For this review, take the finished solid that the model builds, in its own axes (mm). Face numbers are marked on the shaded views. A direction names the side the tool comes from. Give positions to 0.01 mm unless a question says otherwise; leave off trailing zeros. Write each loop counter-clockwise with the first axis right and the second up, starting at its lowest first coordinate (ties: lowest second). Pieces come first, ordered by that corner, then holes. Notation, with made-up numbers: (-37.5, 3) -> (17.5, 3) arc R26 ccw to (17.5, 41) -> close; hole circle Ø6 at (43, 84). An arc over 180 degrees is marked (long way). Return JSON: item names as keys, results as strings.
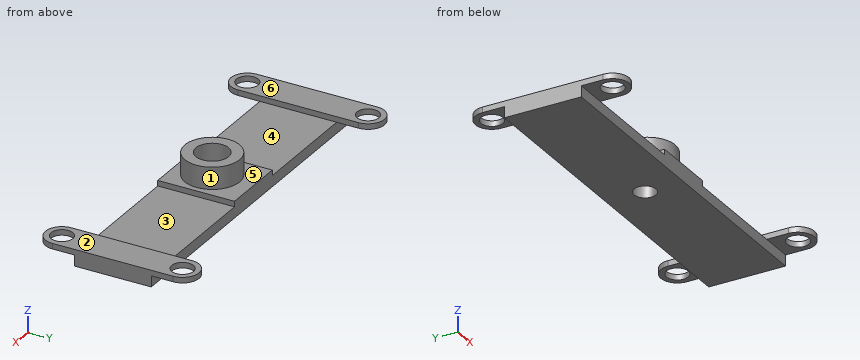
from build123d import *

# Parameters (mm, degrees)
ESBO_O1_W                = 65
ESBO_O1_H                = 14
ESBO_O1_R                = 2
RESSALTO_EXTRUS_O1_DEPTH = 2
ESBO_O2_W                = 12
ESBO_O2_H                = 14
ESBO_O2_R                = 2
RESSALTO_EXTRUS_O2_DEPTH = 1
ESBO_O3_R                = 5
ESBO_O3_R_2              = 3
RESSALTO_EXTRUS_O3_DEPTH = 4


with BuildPart() as part:
    # Esboço1 → Ressalto-extrusão1 (new body)
    with BuildSketch(Plane.XY):
        with Locations((-6.935469367, 10.321486594)):
            Rectangle(ESBO_O1_W, ESBO_O1_H)
        with Locations((-6.935469367, 10.321486594)):
            Circle(ESBO_O1_R, mode=Mode.SUBTRACT)
    extrude(amount=RESSALTO_EXTRUS_O1_DEPTH)

    # Esboço2 → Ressalto-extrusão2 (add)
    # profile 1 of 3: a face of its own
    with BuildSketch(Plane.XY.offset(2)):
        with Locations((-6.935469367, 10.321486594)):
            Rectangle(ESBO_O2_W, ESBO_O2_H)
        with Locations((-6.935469367, 10.321486594)):
            Circle(ESBO_O2_R, mode=Mode.SUBTRACT)
    # profile 2 of 3: a face of its own
    with BuildSketch(Plane.XY.offset(2)):
        with BuildLine():
            Line((-33.435469367, 21.321486594), (-33.435469367, -0.678513406))
            ThreePointArc((-33.435469367, -0.678513406), (-36.435469367, -3.678513406), (-39.435469367, -0.678513406))
            Line((-39.435469367, -0.678513406), (-39.435469367, 21.321486594))
            ThreePointArc((-39.435469367, 21.321486594), (-36.435469367, 24.321486594), (-33.435469367, 21.321486594))
        make_face()
        with Locations((-36.435469367, 21.321486594)):
            Circle(ESBO_O2_R, mode=Mode.SUBTRACT)
        with Locations((-36.435469367, -0.678513406)):
            Circle(ESBO_O2_R, mode=Mode.SUBTRACT)
    # profile 3 of 3: a face of its own
    with BuildSketch(Plane.XY.offset(2)):
        with BuildLine():
            Line((25.564530633, 21.321486594), (25.564530633, -0.678513406))
            ThreePointArc((25.564530633, -0.678513406), (22.564530633, -3.678513406), (19.564530633, -0.678513406))
            Line((19.564530633, -0.678513406), (19.564530633, 21.321486594))
            ThreePointArc((19.564530633, 21.321486594), (22.564530633, 24.321486594), (25.564530633, 21.321486594))
        make_face()
        with Locations((22.564530633, -0.678513406)):
            Circle(ESBO_O2_R, mode=Mode.SUBTRACT)
        with Locations((22.564530633, 21.321486594)):
            Circle(ESBO_O2_R, mode=Mode.SUBTRACT)
    extrude(amount=RESSALTO_EXTRUS_O2_DEPTH)

    # Esboço3 → Ressalto-extrusão3 (add)
    with BuildSketch(Plane.XY.offset(3)):
        with Locations((-6.935469367, 9.821486594)):
            Circle(ESBO_O3_R)
        with Locations((-6.935469367, 9.821486594)):
            Circle(ESBO_O3_R_2, mode=Mode.SUBTRACT)
    extrude(amount=RESSALTO_EXTRUS_O3_DEPTH)


solid = part.part
1. The part is to be moulded in two halves that separate along X. For the marked faces 1, 2 and 3, say which applies: +X half, -X half, draft (parallel to the pull), parting line (faces both ways), or undercut.
Results found:
{"face 1": "parting line", "face 2": "draft", "face 3": "undercut"}
2. To check wall thickness, follow probe 1 along X at (y, z) = (8, 3.5); probe 2 along Y at (x, z) = (-2.5, 0.75); probe 3 along X at (y, z) = (10.75, 5). State the ranges of each line that lie inside material, in increasing order.
Results found:
{"probe 1": "x = -11.59 to -9.32, -4.55 to -2.28", "probe 2": "y = 3.32 to 17.32", "probe 3": "x = -11.85 to -9.79, -4.08 to -2.02"}
3. Add section B-B, the plane x = -7. State the section outline as (y, z) points.
Results found:
{"outline": "(3.32, 0) -> (8.32, 0) -> (8.32, 3) -> (6.82, 3) -> (6.82, 7) -> (4.82, 7) -> (4.82, 3) -> (3.32, 3) -> close; (12.32, 0) -> (17.32, 0) -> (17.32, 3) -> (14.82, 3) -> (14.82, 7) -> (12.82, 7) -> (12.82, 3) -> (12.32, 3) -> close"}
4. For the marked faces 4, 5 and 6, list the 3-axis set-ups (+Z, -Z, +X, -X, +Y, -Y) from which the entire face can be reached by the end or side of a thin tool; tool diameter is ignored.
Results found:
{"face 4": "+Z, +Y, -Y", "face 5": "+Z", "face 6": "+Z, -X, +Y, -Y"}
5. Add section A-A, the plane y = 4. State the section outline as (x, z) points.
Results found:
{"outline": "(-39.44, 0) -> (25.56, 0) -> (25.56, 3) -> (19.56, 3) -> (19.56, 2) -> (-0.94, 2) -> (-0.94, 3) -> (-12.94, 3) -> (-12.94, 2) -> (-33.44, 2) -> (-33.44, 3) -> (-39.44, 3) -> close"}
6. For pin 1 (3 mm diameter, centred on x = -35.5, y = 15, fed in from +Z); pin 2 (3.5 mm diameter, centred on x = 6.5, z = 1, fed in from -Y); pin 3 (3 mm diameter, centred on x = 23.5, y = 20, fed in from -Z), all flat-tipped, find the tip position at first contact; note any pin that passes through.
Results found:
{"pin 1": "stops at z = 3", "pin 2": "stops at y = 3.32", "pin 3": "stops at z = 2"}
7. Add section D-D, the plane z = 1.25. State the section outline as (x, y) points, plus the area to 3 significant figures.
Results found:
{"outline": "(-39.44, 3.32) -> (25.56, 3.32) -> (25.56, 17.32) -> (-39.44, 17.32) -> close; hole circle Ø4 at (-6.94, 10.32)", "area": "897 mm²"}
8. Add section C-C, the plane y = 20.25. State the section outline as (x, z) points, plus the area to 3 significant figures.
Results found:
{"outline": "(-39.44, 2) -> (-38.12, 2) -> (-38.12, 3) -> (-39.44, 3) -> close; (-34.75, 2) -> (-33.44, 2) -> (-33.44, 3) -> (-34.75, 3) -> close; (19.56, 2) -> (20.88, 2) -> (20.88, 3) -> (19.56, 3) -> close; (24.25, 2) -> (25.56, 2) -> (25.56, 3) -> (24.25, 3) -> close", "area": "5.24 mm²"}
